Geometry: final body of the model. Coordinates: model frame, mm. A direction names the side the tool comes from. Give positions to 0.01 mm unless a question says otherwise; leave off trailing zeros. Write each loop counter-clockwise with the first axis right and the second up, starting at its lowest first coordinate (ties: lowest second). Pieces come first, ordered by that corner, then holes. Notation, with made-up numbers: (-30, -7) - (-24, -7) arc R15 ccw to (-24, 11) - close; hole circle Ø3 at (39.5, 63.5). An arc over 180 degrees is marked (long way). Use CSV: the item, a comma, the result in double quotes. Start each with the question number.
(1) Section B-B on x = 0. Output: boundary loops of the cut face in (y, z) (3 decimals), and give its area (3 significant figures).
(2) Section A-A on y = 10. Output: boundary loops of the cut face in (x, z) (3 decimals).
(3) Reachability of faces 1 (the flat face through (-31.5, 7.6, -20.447)), 2 (the flat face through (21.082, 28, -1)), 3 (the cylindrical face through (32.28, 9.04, -22.33)), 4 (the flat face through (-30, 20, -22)), 5 (the flat face through (30, 20, -22)) from +Z, -Z, +X, -X, +Y, -Y: full face, straight path, thin tool, end or side. Return the list, or none.
(4) Section D-D on z = -7.5. Output: boundary loops of the cut face in (x, y).
(5) Section C-C on z = -2. Output: boundary loops of the cut face in (x, y).
(6) Draft query along X for faces 6 (the flat face through (-36.322, 10, -22)), 7 (the flat face through (28, 8, -20.447)), 8 (the flat face through (-5, 20, -2)). Return one class per face: released by +X, released by -X, zero draft, split by the parting line, or undercut.
(7) First-contact query: pin 1 Ø12 at (y, z) = (8.5, -8.5) entering from +X; pin 2 Ø7.5 at (y, z) = (28.5, 2.5) entering from -X; pin 3 Ø4.5 at (x, y) = (-29.972, 10) entering from -Z; pin 4 Ø4 at (x, z) = (-27.5, -21.5) entering from +Y. Flat tips, straight axial feed; report the tip coordinate or a pass-through.
(8) Line query: probe 1 along X at (y, z) = (25, 20.5); probe 2 along Z at (x, y) = (0, 11.75) (3 decimals); probe 3 along Z at (x, y) = (-6, 27). Output: solid intervals per line, ascending. Write a range as [from, to].
from build123d import *

# Parameters (mm, degrees)
BOSS_EXTRUDE1_DEPTH = 20
BOSS_EXTRUDE2_DEPTH = 15.24
SKETCH3_R           = 2.5
CUT_EXTRUDE1_DEPTH  = 4.81
SKETCH4_R           = 5.08
CUT_EXTRUDE2_DEPTH  = 21


with BuildPart() as part:
    # Sketch1 → Boss-Extrude1 (new body)
    with BuildSketch(Plane(origin=(0, 0, 0), x_dir=(1, 0, 0), z_dir=(0, 1, 0))):
        Polygon((-23.622, -24.257), (23.622, -24.257), (23.622, 20.447), (36.322, 20.447), (36.322, 24.257), (23.622, 24.257), (-23.622, 24.257), (-36.322, 24.257), (-36.322, 20.447), (-23.622, 20.447), align=None)
    extrude(amount=BOSS_EXTRUDE1_DEPTH)

    # Sketch2 → Boss-Extrude2 (add)
    with BuildSketch(Plane(origin=(0, 20, 0), x_dir=(1, 0, 0), z_dir=(0, 1, 0))):
        Polygon((-23.622, 24.257), (-21.082, 24.257), (-21.082, -21.717), (21.082, -21.717), (21.082, 24.257), (23.622, 24.257), (23.622, -24.257), (-21.668534476, -24.257), (-23.622, -24.257), align=None)
    extrude(amount=BOSS_EXTRUDE2_DEPTH)

    # Sketch3 → Cut-Extrude1 (cut, through all)
    with BuildSketch(Plane.XY.offset(-20.447)):
        with Locations((29.972, 10)):
            Circle(SKETCH3_R)
    cut_extrude1 = extrude(amount=-CUT_EXTRUDE1_DEPTH, mode=Mode.SUBTRACT)

    # Mirror1: Cut-Extrude1 across plane
    add(cut_extrude1.mirror(Plane(origin=(0, 0, 0), x_dir=(0, 0, 1), z_dir=(1, 0, 0))), mode=Mode.SUBTRACT)

    # Sketch4 → Cut-Extrude2 (cut, through all)
    with BuildSketch(Plane(origin=(0, 20, 0), x_dir=(1, 0, 0), z_dir=(0, 1, 0))):
        with Locations((0, -0.635)):
            Circle(SKETCH4_R)
    extrude(amount=-CUT_EXTRUDE2_DEPTH, mode=Mode.SUBTRACT)


solid = part.part
Check values:
1,outline,"(0, -24.257) - (20, -24.257) - (20, -4.445) - (0, -4.445) - close; (0, 5.715) - (20, 5.715) - (20, 21.717) - (35.24, 21.717) - (35.24, 24.257) - (0, 24.257) - close"
1,area,"806 mm²"
2,outline,"(-36.322, -24.257) - (-32.472, -24.257) - (-32.472, -20.447) - (-36.322, -20.447) - close; (-27.472, -24.257) - (27.472, -24.257) - (27.472, -20.447) - (23.622, -20.447) - (23.622, 24.257) - (-23.622, 24.257) - (-23.622, -20.447) - (-27.472, -20.447) - close; (32.472, -24.257) - (36.322, -24.257) - (36.322, -20.447) - (32.472, -20.447) - close; hole circle Ø10.16 at (0, 0.635)"
3,face 1,"+Z, -X, +Y, -Y"
3,face 2,"-Z, +Y"
3,face 3,"+Z, -Z"
3,face 4,"+Z, -Z, -X, +Y"
3,face 5,"+Z, -Z, +X, +Y"
4,outline,"(-23.62, 0) - (23.62, 0) - (23.62, 35.24) - (21.08, 35.24) - (21.08, 20) - (-21.08, 20) - (-21.08, 35.24) - (-23.62, 35.24) - close"
5,outline,"(-23.62, 0) - (-4.34, 0) - (-4.34, 20) - (-21.08, 20) - (-21.08, 35.24) - (-23.62, 35.24) - close; (4.34, 0) - (23.62, 0) - (23.62, 35.24) - (21.08, 35.24) - (21.08, 20) - (4.34, 20) - close"
6,face 6,"released by -X"
6,face 7,"zero draft"
6,face 8,"undercut"
7,pin 1,"stops at x = 23.62"
7,pin 2,"stops at x = -23.62"
7,pin 3,"passes through"
7,pin 4,"stops at y = 20"
8,probe 1,"x = [-23.62, -21.08], [21.08, 23.62]"
8,probe 2,"z = [-24.257, -4.445], [5.715, 24.257]"
8,probe 3,"z = [21.72, 24.26]"
